Source: CAD feature listing. Evaluate the final solid. Frame: model axes, mm. A direction names the side the tool comes from. Coordinates: 2 decimals unless noted, no trailing zeros. Loops run counter-clockwise (first coordinate to the right, second up) from the corner with the lowest first, then second, coordinate; pieces in that order, holes last. Notation, with made-up numbers: (55.25, 53.25) -> (111.25, 53.25) arc R17 cw to (111.25, 70.25) -> close; hole circle Ø5 at (76, 80.25). An arc over 180 degrees is marked (long way). Answer as a JSON object with one key per item and string values. Group by question number.
Autodesk Inventor part; units mm, degrees
ref_plane "YZ Plane" through (0, 0, 0) normal (1, 0, 0) x (0, 1, 0)
ref_plane "XZ Plane" through (0, 0, 0) normal (0, 1, 0) x (-1, 0, 0)
ref_plane "XY Plane" through (0, 0, 0) normal (0, 0, 1) x (1, 0, 0)
sketch "Sketch1" plane through (0, 0, 0) normal (0, 0, 1) x (1, 0, 0)
  line L0 (-31, -31) -> (31, -31)
  line L1 (31, -31) -> (31, 31)
  line L2 (31, 31) -> (-31, 31)
  line L3 (-31, 31) -> (-31, -31)
  line L4 (-31, -31) -> (31, 31) construction
  line L5 (31, -31) -> (-31, 31) construction
  line L6 (-33, 33) -> (33, 33)
  line L7 (33, 33) -> (33, -33)
  line L8 (33, -33) -> (-33, -33)
  line L9 (-33, -33) -> (-33, 33)
  point P0 (0, 0)
  dimension "d0" = 62
  dimension "d1" = 62
  dimension "d2" = 2
extrude "Extrusion1" add sketch "Sketch1" along normal blind 2 contours L3 L2 L1 L0 | L6 L7 L8 L9
extrude "Extrusion2" add sketch "Sketch1" against normal blind 12
sketch "Sketch2" plane through (-33, 33, 2) normal (0, 1, 0) x (1, 0, 0)
  line L0 (13, 3) -> (53, 3)
  line L1 (53, 3) -> (53, 0)
  line L2 (53, 0) -> (13, 0)
  line L3 (13, 0) -> (13, 3)
  line L4 (0, 14) -> (0, 0)
  line L5 (0, 14) -> (66, 14)
  point P0 (33, 2)
  dimension "d7" = 40
  dimension "d8" = 3
  dimension "d9" = 13
  dimension "d10" = 11
extrude "Extrusion3" add sketch "Sketch2" along normal blind 12
sketch "Sketch3" plane through (20, 33, -1) normal (0, 0, -1) x (-1, 0, 0)
  line L0 (40, 12) -> (0, 12)
  line L1 (40, 0) -> (40, 12)
  line L2 (0, 12) -> (40, 12)
  line L3 (40, 12) -> (40, 9)
  line L4 (40, 9) -> (0, 9)
  line L5 (0, 9) -> (0, 12)
  point P0 (20, -33)
  dimension "d13" = 3
extrude "Extrusion4" add sketch "Sketch3" along normal blind 80
sketch "Sketch4" plane through (-20, 42, -1) normal (0, -1, 0) x (1, 0, 0)
  line L0 (30.5, -63) -> (9.5, -63)
  line L1 (9.5, -63) -> (9.5, -22)
  line L2 (9.5, -22) -> (30.5, -22)
  line L3 (30.5, -22) -> (30.5, -63)
  line L4 (40, 3) -> (40, -80)
  line L5 (0, 3) -> (40, 3)
  point P0 (20, 1)
  dimension "d16" = 21
  dimension "d17" = 41
  dimension "d18" = 9.5
  dimension "d19" = 25
extrude "Extrusion5" cut sketch "Sketch4" against normal blind 80
sketch "Sketch5" plane through (-20, 42, -1) normal (0, -1, 0) x (1, 0, 0)
  line L0 (30.5, -63) -> (9.5, -63)
  line L1 (30.5, -63) -> (9.5, -63)
  line L2 (9.5, -63) -> (9.5, -70)
  line L3 (9.5, -70) -> (30.5, -70)
  line L4 (30.5, -70) -> (30.5, -63)
  circle A0 centre (15, -66.75) radius 2.25
  line L5 (30.5, -22) -> (30.5, -63)
  line L6 (30.5, -22) -> (9.5, -22)
  line L7 (9.5, -22) -> (9.5, -15)
  line L8 (9.5, -15) -> (30.5, -15)
  line L9 (30.5, -15) -> (30.5, -22)
  circle A1 centre (25, -18.25) radius 2.25
  point P0 (20, 1)
  point P1 (15.4717, -69.81)
  point P2 (14.5283, -69.81)
  point P3 (24.5283, -15.19)
  point P4 (25.4717, -15.19)
  dimension "d22" = 7
  dimension "d23" = 4.5
  dimension "d24" = 3.75
  dimension "d25" = 5.5
  dimension "d26" = 7
  dimension "d27" = 4.5
  dimension "d28" = 5.5
  dimension "d29" = 3.75
extrude "Extrusion6" cut sketch "Sketch5" against normal blind 80 contours A0 | A1
sketch "Sketch6" plane through (-33, -33, 2) normal (0, -1, 0) x (1, 0, 0)
  line L0 (0, 0) -> (66, 0)
  line L1 (66, -14) -> (0, -14)
  line L2 (0, 0) -> (66, 0)
  line L3 (66, 0) -> (66, -14)
  line L4 (66, -14) -> (0, -14)
  line L5 (0, -14) -> (0, 0)
  point P0 (33, -2)
extrude "Extrusion7" cut sketch "Sketch6" against normal up to surface (75 mm away)
sketch "Sketch7" plane through (-20, 42, -81) normal (0, -1, 0) x (1, 0, 0)
  line L0 (40, 83) -> (40, 0)
  line L1 (40, 0) -> (85, 0)
  line L2 (85, 0) -> (85, 83)
  line L3 (85, 83) -> (40, 83)
  line L4 (40, 83) -> (40, 0)
  line L5 (85, 33) -> (40, 33)
  point P0 (20, 81)
  point P1 (40, 33)
  dimension "d34" = 45
  dimension "d35" = 83
  dimension "d36" = 50
extrude "Extrusion8" add sketch "Sketch7" against normal up to surface (3 mm away) contours L3 L2 L5 L0
sketch "Sketch8" plane through (-20, 42, -81) normal (0, -1, 0) x (1, 0, 0)
  line L0 (0, 83) -> (85, 83)
  line L1 (85, 83) -> (85, 0)
  line L2 (85, 0) -> (0, 0)
  line L3 (0, 0) -> (0, 83)
  line L4 (85, 7) -> (0, 7)
  line L5 (85, 33) -> (85, 83)
  line L6 (-12.2623, 85.093) -> (0, 83)
  line L7 (0, 83) -> (-11.5686, 87.0435)
  line L8 (-11.5686, 87.0435) -> (85, 70.5603)
  line L9 (0, 83) -> (100, 83)
  line L10 (100, 83) -> (100, 68)
  line L11 (100, 68) -> (0, 68)
  line L12 (0, 68) -> (0, 83)
  point P0 (20, 81)
  point P1 (0, 73.8499)
  point P2 (27.25, 61.75)
  point P3 (27.25, 61.75)
  point P4 (25.55, 64.81)
  point P5 (0, 68)
  point P6 (85, 68)
  dimension "d40" = 83
  dimension "d41" = 7
  dimension "d43" = 15
extrude "Extrusion9" cut sketch "Sketch8" against normal blind 10 contours L0 L8 L1 L11 L3 | L0 L1 L8 | L4 L1 L2 L3
sketch "Sketch9" plane through (20, 42, -48) normal (0, -1, 0) x (1, 0, 0)
  line L0 (45, 0) -> (45, 35)
  line L1 (0, 0) -> (45, 0)
  line L2 (45, 35) -> (42, 35)
  line L3 (42, 35) -> (42, 0)
  line L4 (42, 0) -> (45, 0)
  line L5 (45, 0) -> (45, 35)
  point P0 (-20, 48)
  dimension "d46" = 3
extrude "Extrusion10" add sketch "Sketch9" along normal blind 100
sketch "Sketch10" plane through (65, 45, -13) normal (1, 0, 0) x (0, 0, -1)
  circle A0 centre (18, -56.25) radius 2.125
  circle A1 centre (18, -93) radius 2.125
  circle A2 centre (18, -74.625) radius 6.45
  line L0 (20.093, -55.8824) -> (22.589, -70.0925)
  line L1 (15.9065, -55.8857) -> (13.439, -70.0643)
  line L2 (20.0935, -93.3643) -> (22.561, -79.1857)
  line L3 (15.8877, -93.2317) -> (13.411, -79.1575)
  line L4 (18, -56.25) -> (18, -74.625)
  line L5 (18, -74.625) -> (18, -93)
  line L6 (35, 0) -> (35, -103)
  line L7 (35, -103) -> (0, -103)
  point P0 (-13, -45)
  dimension "d49" = 4.25
  dimension "d50" = 4.25
  dimension "d51" = 12.9
  dimension "d52" = 9.15
  dimension "d53" = 9.15
  dimension "d54" = 41
  dimension "d57" = 17
  dimension "d58" = 10
extrude "Extrusion11" cut sketch "Sketch10" against normal blind 2.5
properties part number "pan_base_holder_v1"
1. Section query B-B on z = -19.25. Return loops of the section in (x, y).
2. Mould query, pull axis X, two halves, no side actions, for faces 1 (the face through (65, -6, -31)), 2 (the face through (0, 43, -23)), 3 (the face through (-5, 43, -70)), 4 (the face through (63.768, -41.293, -27.667)). Classes: pulls with the +X half, pulls with the -X half, needs draft (parallel to the pull), parting line crosses it, or undercut.
3. Section query A-A on x = -5. Return loops of the section in (y, z).
4. Section query C-C on y = -32. Return loops of the section in (x, z), then the cut area to 3 significant figures.
5. Reachability of faces 5 (the face through (63.77, -41.37, -34.31)), 6 (the face through (62, -7, -30)), 7 (the face through (-10.5, 43, -44)), 8 (the face through (20, 43, -61)) from +Z, -Z, +X, -X, +Y, -Y: full face, straight path, thin tool, end or side. Return the list, or none.
6. Section query D-D on z = -67.75. Return loops of the section in (x, y).
7. Pin query (flat end, axial travel): pin 1 Ø1 at (y, z) = (-45, -49.5) entering from +X; pin 2 Ø4 at (y, z) = (-32, -33) entering from +X; pin 3 Ø17.5 at (y, z) = (15, -34) entering from -X; pin 4 Ø0.9 at (y, z) = (43, -67) entering from +X. Return the tip coordinate at first contact, or that it passes through.
8. Ray query, L1, parallel to Z at x = 5, y = 44.1; L2, parallel to Z at x = -5, y = 44; L3, parallel to X at y = 43, z = -19. Return the intervals inside material, ascending.
Solved:
{
 "1": {"outline": "(-20, 42) -> (2.75, 42) -> (2.75, 45) -> (-20, 45) -> close; (7.25, 42) -> (62, 42) -> (62, -58) -> (65, -58) -> (65, 45) -> (7.25, 45) -> close"},
 "2": {"face 1": "pulls with the +X half", "face 2": "undercut", "face 3": "undercut", "face 4": "needs draft"},
 "3": {"outline": "(42, -74) -> (45, -74) -> (45, -70) -> (42, -70) -> close; (42, -65.5) -> (45, -65.5) -> (45, -64) -> (42, -64) -> close; (42, -23) -> (45, -23) -> (45, -13) -> (42, -13) -> close"},
 "4": {"outline": "(62, -48) -> (65, -48) -> (65, -37) -> (62.5, -37) -> (62.5, -25) -> (65, -25) -> (65, -13) -> (62, -13) -> close", "area": "75.0 mm^2"},
 "5": {"face 5": "+X", "face 6": "+Z, -Z, -X, -Y", "face 7": "+Y, -Y", "face 8": "-Z, +X, +Y, -Y"},
 "6": {"outline": "(-20, 42) -> (-7.25, 42) -> (-7.25, 45) -> (-20, 45) -> close; (-2.75, 42) -> (20, 42) -> (20, 45) -> (-2.75, 45) -> close"},
 "7": {"pin 1": "through", "pin 2": "x = 62.5", "pin 3": "x = 62", "pin 4": "x = 20"},
 "8": {"L1": "-74 to -64, -23 to -21.5, -17 to -13", "L2": "-74 to -70, -65.5 to -64, -23 to -13", "L3": "-20 to 2.76, 7.24 to 65"}
}
